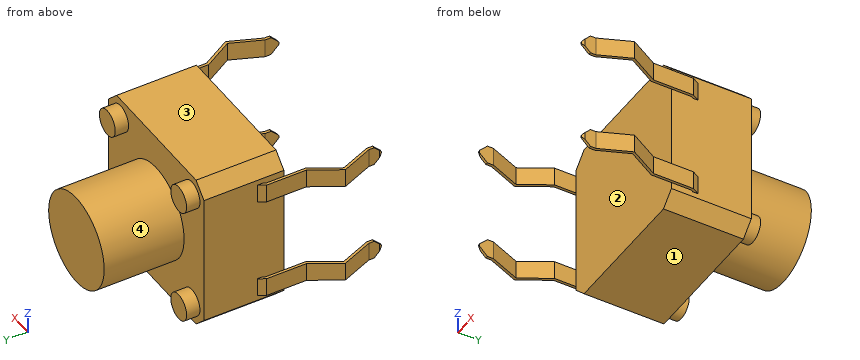
```python
from build123d import *

# Parameters (mm, degrees)
SKETCH1_W               = 6.01
SKETCH1_H               = 6.01
BOSS_EXTRUDE1_DEPTH     = 3
CHAMFER1_SIZE           = 0.5
SKETCH3_R               = 1.75
BOSS_EXTRUDE2_DEPTH     = 3
SKETCH4_R               = 0.5
BOSS_EXTRUDE6_DEPTH     = 0.5
SKETCH5_R               = 0.5
BOSS_EXTRUDE7_DEPTH     = 0.5
SKETCH6_W               = 0.7
SKETCH6_H               = 0.2
MIRROR2_COPY_1_SKETCH_W = 0.7
MIRROR2_COPY_1_SKETCH_H = 0.2
CUT_EXTRUDE1_DEPTH      = 4.782799277


with BuildPart() as part:
    # Sketch1 → Boss-Extrude1 (new body)
    with BuildSketch(Plane(origin=(0, 0, 0), x_dir=(1, 0, 0), z_dir=(0, 1, 0))):
        Rectangle(SKETCH1_W, SKETCH1_H)
    extrude(amount=BOSS_EXTRUDE1_DEPTH)

    # Chamfer1
    chamfer1_edges = [part.edges().sort_by_distance(p)[0] for p in [
        (3.005, 1.5, 3.005),
        (-3.005, 1.5, 3.005),
        (-3.005, 1.5, -3.005),
        (3.005, 1.5, -3.005),
    ]]
    chamfer(chamfer1_edges, length=CHAMFER1_SIZE)

    # Sketch3 → Boss-Extrude2 (add)
    with BuildSketch(Plane(origin=(0, 3, 0), x_dir=(1, 0, 0), z_dir=(0, 1, 0))):
        Circle(SKETCH3_R)
    extrude(amount=BOSS_EXTRUDE2_DEPTH)

    # Sketch4 → Boss-Extrude6 (add)
    with BuildSketch(Plane(origin=(0, 3, 0), x_dir=(1, 0, 0), z_dir=(0, 1, 0))):
        with Locations((2.25, 2.25)):
            Circle(SKETCH4_R)
        with Locations((2.25, -2.25)):
            Circle(SKETCH4_R)
        with Locations((-2.25, 2.25)):
            Circle(SKETCH4_R)
    extrude(amount=BOSS_EXTRUDE6_DEPTH)

    # Sketch5 → Boss-Extrude7 (add)
    with BuildSketch(Plane(origin=(0, 3, 0), x_dir=(1, 0, 0), z_dir=(0, 1, 0))):
        with Locations((-2.25, -2.25)):
            Circle(SKETCH5_R)
    extrude(amount=BOSS_EXTRUDE7_DEPTH)

    # Sweep1: sweep along a path in Sketch7
    with BuildLine(Plane.XY) as sweep1_path:
        Line((-3.005, 0.9), (-3.105, 0.726794919))
        Line((-3.105, 0.726794919), (-3.105, -0.773205081))
        Line((-3.105, -0.773205081), (-3.72715614, -1.850811126))
        Line((-3.72715614, -1.850811126), (-3.25, -3))
        Line((-3.25, -3), (-3.25, -3.5))
    # Sketch6 → Sweep1 (sweep)
    with BuildSketch(Plane.ZY.offset(3.005)):
        with Locations((-1.955, 0.9)):
            Rectangle(SKETCH6_W, SKETCH6_H)
    sweep1 = sweep(path=sweep1_path.line, transition=Transition.RIGHT)

    # Mirror1: Sweep1 across plane
    add(sweep1.mirror(Plane.XY))

    # Mirror2: Sweep1 across plane
    add(sweep1.mirror(Plane(origin=(0, 0, 0), x_dir=(0, 0, 1), z_dir=(1, 0, 0))))

    # Mirror2 copy 1: sweep along a path in Mirror2 copy 1 path
    with BuildLine(Plane(origin=(0, 0, 0), x_dir=(-1, 0, 0), z_dir=(0, 0, -1))) as mirror2_copy_1_path:
        Line((-3.005, 0.9), (-3.105, 0.726794919))
        Line((-3.105, 0.726794919), (-3.105, -0.773205081))
        Line((-3.105, -0.773205081), (-3.72715614, -1.850811126))
        Line((-3.72715614, -1.850811126), (-3.25, -3))
        Line((-3.25, -3), (-3.25, -3.5))
    # Mirror2 copy 1 sketch → Mirror2 copy 1 (sweep)
    with BuildSketch(Plane(origin=(3.005, 0, 0), x_dir=(0, 0, -1), z_dir=(1, 0, 0))):
        with Locations((-1.955, 0.9)):
            Rectangle(MIRROR2_COPY_1_SKETCH_W, MIRROR2_COPY_1_SKETCH_H)
    sweep(path=mirror2_copy_1_path.line, transition=Transition.RIGHT)

    # Sketch8 → Cut-Extrude1 (cut, symmetric)
    with BuildSketch(Plane(origin=(0, 0, 0), x_dir=(0, 0, -1), z_dir=(1, 0, 0))):
        with BuildLine():
            Line((-2.305, -3.211682602), (-2.305, -3.58660254))
            Line((-2.305, -3.58660254), (-1.605, -3.58660254))
            Line((-1.605, -3.58660254), (-1.605, -3.211682602))
            Line((-1.605, -3.211682602), (-1.881694927, -3.48928466))
            ThreePointArc((-1.881694927, -3.48928466), (-1.952077784, -3.518688814), (-2.022718654, -3.489910032))
            Line((-2.022718654, -3.489910032), (-2.305, -3.211682602))
        make_face()
    cut_extrude1 = extrude(amount=CUT_EXTRUDE1_DEPTH, both=True, mode=Mode.SUBTRACT)

    # Mirror3: Cut-Extrude1 across plane
    add(cut_extrude1.mirror(Plane.XY), mode=Mode.SUBTRACT)


solid = part.part
```
Check sheet for the modelled part. Datum: model origin and axes. Units: mm. Face numbers are marked on the shaded views. A direction names the side the tool comes from. Round coordinates to 2 decimals unless told otherwise and drop trailing zeros. Loops run counter-clockwise (first coordinate to the right, second up) from the corner with the lowest first, then second, coordinate; pieces in that order, holes last. Notation, with made-up numbers: (-38.5, 75.25) -> (-4.5, 75.25) arc R13 cw to (-4.5, 99.25) -> close; hole circle Ø7 at (-29.5, -33.75). An arc over 180 degrees is marked (long way). Write item = value, one per line. Start each with the question number.
1) Thickness scan on probe 1 along Y at (x, z) = (-2.5, -2.5); probe 2 along Y at (x, z) = (0.25, 0.5); probe 3 along X at (y, z) = (2.75, -1.25) (3 decimals). Record the ranges inside material, lowest first.
2) Release check for a two-part mould opening along X. For the marked faces 1 and 2 record: released by +X, released by -X, zero draft, split by the parting line, or undercut.
3) Set-up check for the marked faces 3 and 4: record each of +Z, -Z, +X, -X, +Y, -Y from which the full face is reachable in a straight line by a thin tool's end or side.
4) Sectioned sample at A-A, the plane y = -1.25. Record the cut outline in (x, z) (3 decimals), plus the area to 3 significant figures.
5) Gauge pin test, flat ends, axial feed: pin 1 Ø1.5 at (y, z) = (1.5, -1) entering from -X (3 decimals); pin 2 Ø1.5 at (y, z) = (2, -0.5) entering from +X (3 decimals); pin 3 Ø0.9 at (x, y) = (3.5, 0) entering from +Z (3 decimals). Record the tip position at first contact, or that the pin passes through.
6) Sectioned sample at D-D, the plane y = 2.75. Record the cut outline in (x, z) (3 decimals), plus the area to 3 significant figures.
7) Sectioned sample at B-B, the plane z = 0. Record the cut outline in (x, y) (3 decimals).
8) Sectioned sample at C-C, the plane x = -2.25. Record the cut outline in (y, z) (3 decimals).
Results are:
q1.probe_1 = 0 to 3.5
q1.probe_2 = 0 to 6
q1.probe_3 = -3.005 to 3.005
q2.face_1 = zero draft
q2.face_2 = undercut
q3.face_3 = +Z, +X, -X, +Y, -Y
q3.face_4 = +Y
q4.outline = (-3.438, -2.305) -> (-3.323, -2.305) -> (-3.323, -1.605) -> (-3.438, -1.605) -> close; (-3.438, 1.605) -> (-3.323, 1.605) -> (-3.323, 2.305) -> (-3.438, 2.305) -> close; (3.323, -2.305) -> (3.438, -2.305) -> (3.438, -1.605) -> (3.323, -1.605) -> close; (3.323, 1.605) -> (3.438, 1.605) -> (3.438, 2.305) -> (3.323, 2.305) -> close
q4.area = 0.323 mm^2
q5.pin_1 = -3.005
q5.pin_2 = 3.005
q5.pin_3 = 2.305
q6.outline = (-3.005, -2.505) -> (-2.505, -3.005) -> (2.505, -3.005) -> (3.005, -2.505) -> (3.005, 2.505) -> (2.505, 3.005) -> (-2.505, 3.005) -> (-3.005, 2.505) -> close
q6.area = 35.6 mm^2
q7.outline = (-3.005, 0) -> (3.005, 0) -> (3.005, 3) -> (1.75, 3) -> (1.75, 6) -> (-1.75, 6) -> (-1.75, 3) -> (-3.005, 3) -> close
q8.outline = (0, -3.005) -> (3, -3.005) -> (3, -2.75) -> (3.5, -2.75) -> (3.5, -1.75) -> (3, -1.75) -> (3, 1.75) -> (3.5, 1.75) -> (3.5, 2.75) -> (3, 2.75) -> (3, 3.005) -> (0, 3.005) -> close
